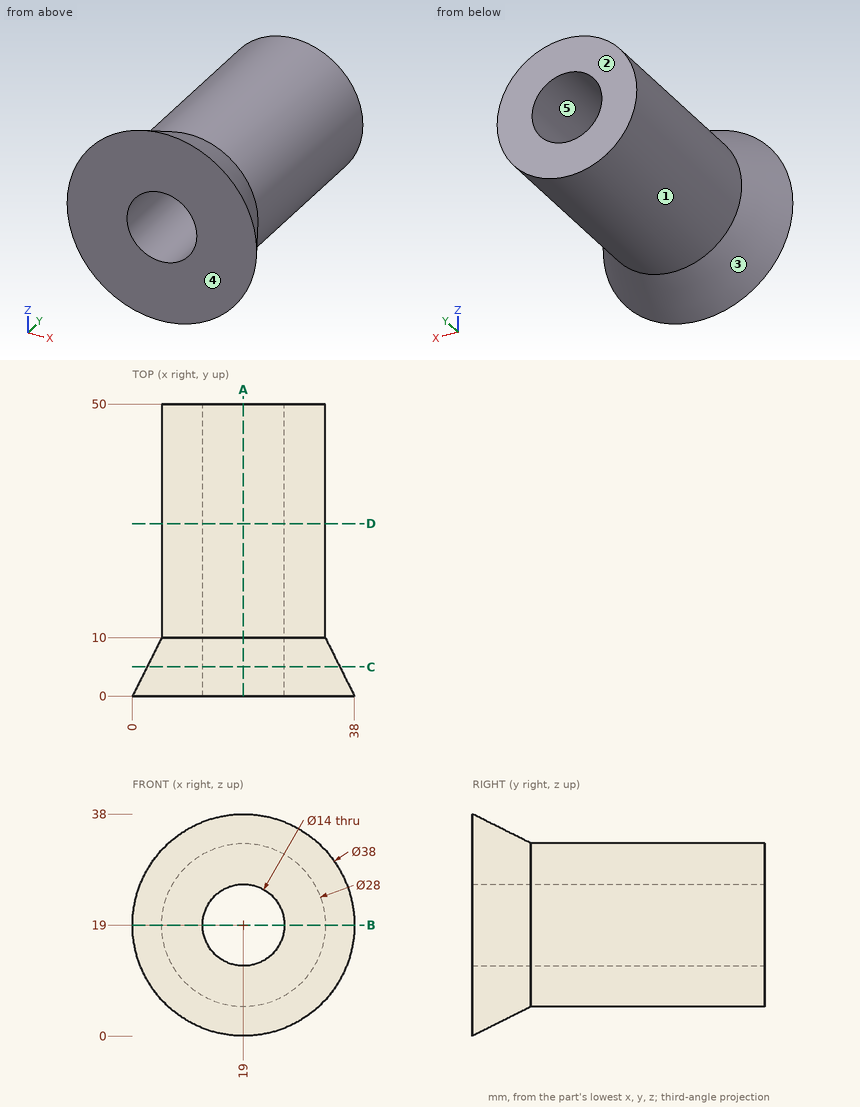
Geometry: see drawing. Coordinates: mm, zero at the bounding-box minimum. A direction names the side the tool comes from. Round coordinates to 2 decimals unless told otherwise and drop trailing zeros. Write each loop counter-clockwise with the first axis right and the second up, starting at its lowest first coordinate (ties: lowest second). Pieces come first, ordered by that corner, then holes.
1) Cut plane C-C (y = 5). Return the cut outline in (x, z).
2) Contact query for flat-ended pins moving along their axis: P1, Ø6, axis at x = 29, y = 9, coming from the +Z side; P2, Ø3, axis at x = 6.5, y = 21, coming from the -Z side; P3, Ø5, axis at x = 32, y = 35.5, coming from the +Z side; P4, Ø12.5, axis at x = 19, z = 19, coming from the +Y side. Output: stop coordinate, or through.
3) Draft query along X for the marked faces 3, 4 and 5. Return one class per face: pulls with the +X half, pulls with the -X half, needs draft (parallel to the pull), parting line crosses it, or undercut.
4) Ray query, L1, parallel to X at y = 21, z = 19; L2, parallel to Z at x = 17.5, y = 12.5. Return the intervals inside material, ascending.
5) Cut plane A-A (x = 19). Return the cut outline in (y, z).
6) Cut plane D-D (y = 29.5). Return the cut outline in (x, z).
7) Cut plane B-B (z = 19). Return the cut outline in (x, y).
8) Reachability of the marked faces 1 and 2 from +Z, -Z, +X, -X, +Y, -Y: full face, straight path, thin tool, end or side. Return the list, or none.
Geometry says:
1. outline: circle Ø33 at (19, 19); hole circle Ø14 at (19, 19)
2. P1: stops at z = 32.42
2. P2: stops at z = 10.34
2. P3: stops at z = 28.26
2. P4: passes through
3. face 3: parting line crosses it
3. face 4: needs draft
3. face 5: undercut
4. L1: x = 5 to 12, 26 to 33
4. L2: z = 5.08 to 12.16, 25.84 to 32.92
5. outline: (0, 0) - (10, 5) - (50, 5) - (50, 12) - (0, 12) - close; (0, 26) - (50, 26) - (50, 33) - (10, 33) - (0, 38) - close
6. outline: circle Ø28 at (19, 19); hole circle Ø14 at (19, 19)
7. outline: (0, 0) - (12, 0) - (12, 50) - (5, 50) - (5, 10) - close; (26, 0) - (38, 0) - (33, 10) - (33, 50) - (26, 50) - close
8. face 1: +Y
8. face 2: +Z, -Z, +X, -X, +Y
